from build123d import *

# Parameters (mm, degrees)
BOSS_EXTRUDE1_DEPTH = 70
SKETCH3_R           = 50
CUT_EXTRUDE1_DEPTH  = 50


with BuildPart() as part:
    # Sketch2 → Boss-Extrude1 (new body)
    with BuildSketch(Plane(origin=(0, 0, 0), x_dir=(1, 0, 0), z_dir=(0, 1, 0))):
        with BuildLine():
            Line((295.019395576, 60), (-94.904260616, 99.491041282))
            ThreePointArc((-94.904260616, 99.491041282), (-204.853283691, 5.044594719), (-104.980604424, -100))
            Line((-104.980604424, -100), (-85.178624226, -98.01980198))
            Line((-85.178624226, -98.01980198), (295.019395576, -60))
            ThreePointArc((295.019395576, -60), (355.019395576, 0), (295.019395576, 60))
        make_face()
    extrude(amount=BOSS_EXTRUDE1_DEPTH)

    # Sketch3 → Cut-Extrude1 (cut)
    with BuildSketch(Plane(origin=(0, 70, 0), x_dir=(1, 0, 0), z_dir=(0, 1, 0))):
        with Locations(Location((-104.980604424, 0, 0), (0, 0, 270))):
            Circle(SKETCH3_R)
        with Locations(Location((295.019395576, 0, 0), (0, 0, 270))):
            Circle(SKETCH3_R)
    extrude(amount=-CUT_EXTRUDE1_DEPTH, mode=Mode.SUBTRACT)


solid = part.part
Part model, mm, in its own coordinate system. A direction names the side the tool comes from. Coordinates: 2 decimals unless noted, no trailing zeros. Write each loop counter-clockwise with the first axis right and the second up, starting at its lowest first coordinate (ties: lowest second). Pieces come first, ordered by that corner, then holes. Notation, with made-up numbers: (-15, 25) - (17, 25) arc R15 cw to (17, 38) - close; hole circle Ø9 at (10, -18). An arc over 180 degrees is marked (long way). Put each result on its own line as item: value.
1. Probe line 1 along X through (y, z) = (61, 0.5); line 2 along X through (y, z) = (50, -42); line 3 along Z through (x, y) = (-137, 57). List the from-to ranges inside material, lowest first. Write a range as [from, to].
Final values:
line 1: x = [-204.98, -154.98], [-54.98, 245.02], [345.02, 355.02]
line 2: x = [-195.73, -132.11], [-77.85, 267.89], [322.15, 337.87]
line 3: z = [-94.74, -38.4], [38.4, 94.74]
2. Flat gauge pins, fed straight in: pin 1 Ø3 at (x, z) = (97, 30.5) entering from -Y; pin 2 Ø1 at (y, z) = (28.5, -52) entering from +X; pin 3 Ø12 at (y, z) = (25, 38.5) entering from -X; pin 4 Ø10 at (x, y) = (171, 51) entering from -Z. Where does each tip first touch, or does it go through?
Final values:
pin 1: stops at y = 0
pin 2: stops at x = 325.8
pin 3: stops at x = -199.55
pin 4: stops at z = -73.07
3. Two-plate mould, pull along Z, no slides. Class faces 3 (the cylindrical face through (344.594, 45.35, -6.509)), 4 (the flat face through (102.79, 34.51, -79.47)), 5 (the cylindrical face through (355.005, 34.51, 1.319)): +Z half, -Z half, draft (parallel to the pull), parting line (faces both ways), or undercut.
Final values:
face 3: undercut
face 4: -Z half
face 5: parting line
4. Band-saw the part on C-C (x = -111). Write the cut outline in (y, z).
Final values:
outline: (0, -99.82) - (70, -99.82) - (70, -49.64) - (20, -49.64) - (20, 49.64) - (70, 49.64) - (70, 99.82) - (0, 99.82) - close
5. 3-axis set-ups, long thin cutter, end or side, ignore diameter. For faces 1 (the flat face through (9, 70, -1)), 2 (the flat face through (-104, 20, -1)): which of +Z, -Z, +X, -X, +Y, -Y reach the whole face in a straight line?
Final values:
face 1: +Z, -Z, +X, -X, +Y
face 2: +Y
6. Band-saw the part on A-A (z = 0). Write the cut outline in (x, y).
Final values:
outline: (-204.98, 0) - (355.02, 0) - (355.02, 70) - (345.02, 70) - (345.02, 20) - (245.02, 20) - (245.02, 70) - (-54.98, 70) - (-54.98, 20) - (-154.98, 20) - (-154.98, 70) - (-204.98, 70) - close
7. Band-saw the part on D-D (x = 118). Write the cut outline in (y, z).
Final values:
outline: (0, -77.93) - (70, -77.93) - (70, 77.7) - (0, 77.7) - close
8. Band-saw the part on B-B (y = 46.5). Write the cut outline in (x, z), then the cut area to 3 significant figures.
Final values:
outline: (-104.98, 100) arc R100 ccw (long way) to (-94.9, -99.49) - (295.02, -60) arc R60 ccw to (295.02, 60) - close; hole circle Ø100 at (-104.98, 0); hole circle Ø100 at (295.02, 0)
area: 69,800 mm²
